Drawing for the job (mm, zero at the part's lowest x, y, z). Coordinates: 2 decimals unless noted, no trailing zeros. Loops run counter-clockwise (first coordinate to the right, second up) from the corner with the lowest first, then second, coordinate; pieces in that order, holes last. Notation, with made-up numbers: (29.25, 20) - (52.25, 20) arc R20 cw to (52.25, 30) - close; hole circle Ø9 at (55.25, 25). An arc over 180 degrees is marked (long way). Put each result on its own line as item: value.
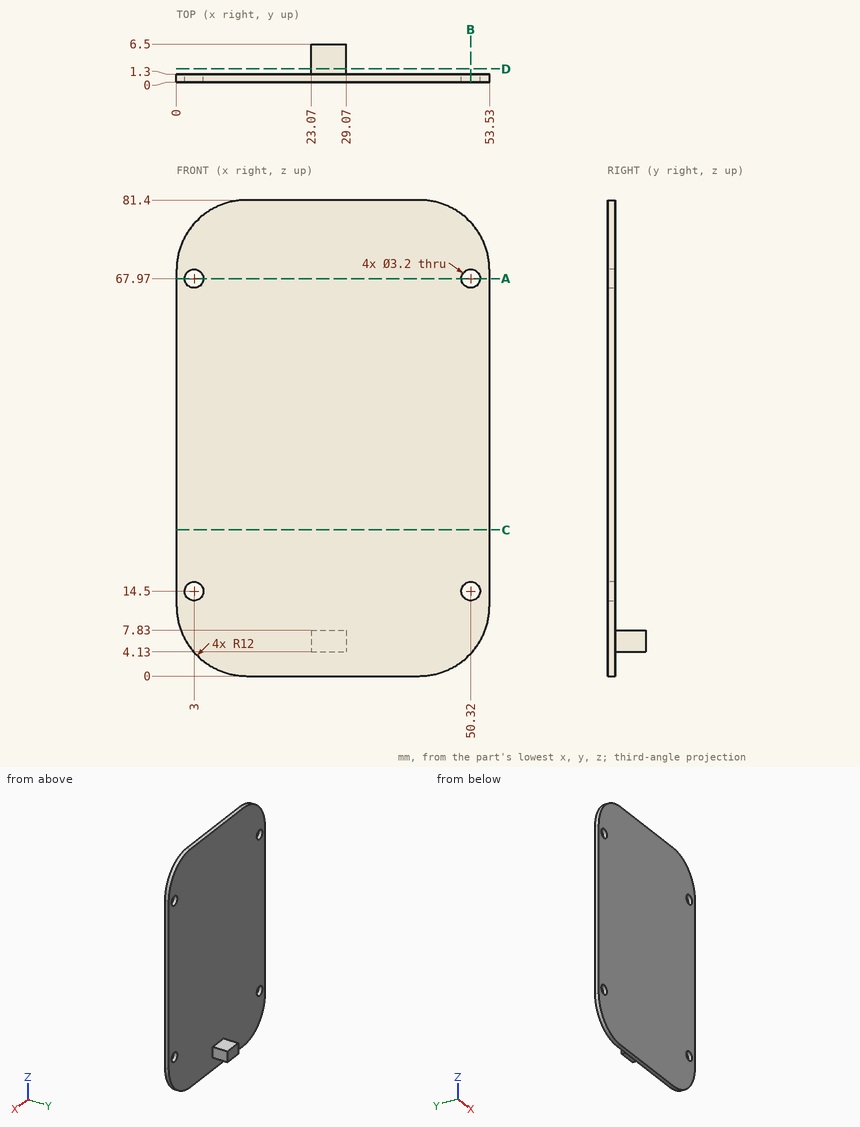
Q1. Pin check, flat tips, straight feed: pin 1 Ø4 at (x, z) = (9, 34.5) entering from +Y; pin 2 Ø1.1 at (y, z) = (5, 6) entering from +X; pin 3 Ø3 at (x, y) = (22.5, 5) entering from +Z. Stop position of each tip, or through.
Determined:
pin 1: y = 1.3
pin 2: x = 29.07
pin 3: z = 7.83
Q2. Wall check: L1, parallel to X at y = 0.8, z = 14.5; L2, parallel to Z at x = 2.5, y = 1; L3, parallel to Y at x = 18, z = 50. Give the ranges that are in metal, low to high. Write a range as from..to.
Determined:
L1: 0..1.4, 4.6..48.72, 51.92..53.53
L2: 4.67..12.98, 16.02..66.45, 69.49..76.73
L3: 0..1.3
Q3. Slice it at D-D, the plane y = 2.25. Give the cut face in (x, z).
Determined:
outline: (23.07, 4.13) - (29.07, 4.13) - (29.07, 7.83) - (23.07, 7.83) - close
Q4. Slice it at A-A, the plane z = 67.97. Give the cut face in (x, y), then the cut area to 3 significant figures.
Determined:
outline: (0, 0) - (1.4, 0) - (1.4, 1.3) - (0, 1.3) - close; (4.6, 0) - (48.72, 0) - (48.72, 1.3) - (4.6, 1.3) - close; (51.92, 0) - (53.53, 0) - (53.53, 1.3) - (51.92, 1.3) - close
area: 61.3 mm2
Q5. Slice it at C-C, the plane z = 25. Give the cut face in (x, y), then the cut area to 3 significant figures.
Determined:
outline: (0, 0) - (53.53, 0) - (53.53, 1.3) - (0, 1.3) - close
area: 69.6 mm2
Q6. Slice it at B-B, the plane x = 50.32. Give the cut face in (y, z).
Determined:
outline: (0, 3.83) - (1.3, 3.83) - (1.3, 12.9) - (0, 12.9) - close; (0, 16.1) - (1.3, 16.1) - (1.3, 66.37) - (0, 66.37) - close; (0, 69.57) - (1.3, 69.57) - (1.3, 77.57) - (0, 77.57) - close
